Input: part model. Units: mm. Frame: model coordinates. Face numbers are marked on the shaded views. Round coordinates to 2 decimals unless told otherwise and drop trailing zeros. Order: outer loops, then holes, each group sorted by start corner. A loop starts at its lowest first (then second) coordinate and runs counter-clockwise, first axis right, second up. Notation, with made-up numbers: (76.25, 21.5) -> (92.25, 21.5) arc R31 ccw to (92.25, 56.5) -> close; hole circle Ø11 at (10, 16). An arc over 180 degrees is marked (long way). Use a Markdown table: item, result.
from build123d import *

# Parameters (mm, degrees)
SKETCH001_R      = 1.5875
EXTRUDE001_DEPTH = 7.62
SKETCH_R         = 3.556
EXTRUDE_DEPTH    = 3.81
BOX_W            = 60.325
BOX_H            = 45.72
BOX_DEPTH        = 6.35
THICKNESS_T      = -2.54
FILLET_R         = 3.56
FILLET001_R      = 6.1


with BuildPart() as extrude001:
    # Sketch001 (on Face9 of Extrude) → Extrude001 (new body)
    with BuildSketch(Plane.XY.offset(6.35)):
        with Locations((6.1, 39.62)):
            Circle(SKETCH001_R)
        with Locations((54.225, 39.62)):
            Circle(SKETCH001_R)
        with Locations((54.225, 6.1)):
            Circle(SKETCH001_R)
        with Locations((6.1, 6.1)):
            Circle(SKETCH001_R)
    extrude(amount=-EXTRUDE001_DEPTH)


with BuildPart() as extrude_body:
    # Sketch (on Face19 of Fillet001) → Extrude (new body)
    with BuildSketch(Plane.XY.offset(2.54)):
        with Locations((6.1, 39.62)):
            Circle(SKETCH_R)
        with Locations((54.225, 39.62)):
            Circle(SKETCH_R)
        with Locations((54.225, 6.1)):
            Circle(SKETCH_R)
        with Locations((6.1, 6.1)):
            Circle(SKETCH_R)
    extrude(amount=EXTRUDE_DEPTH)


with BuildPart() as cut:
    # Box → Box (new body)
    with BuildSketch(Plane.XY):
        with Locations((30.1625, 22.86)):
            Rectangle(BOX_W, BOX_H)
    extrude(amount=BOX_DEPTH)

    # Thickness
    thickness_openings = [cut.faces().sort_by_distance(p)[0] for p in [
        (30.1625, 22.86, 6.35),
    ]]
    offset(amount=THICKNESS_T, openings=thickness_openings, kind=Kind.INTERSECTION)

    # Fillet
    fillet_edges = [cut.edges().sort_by_distance(p)[0] for p in [
        (2.54, 2.54, 4.445),
        (2.54, 43.18, 4.445),
        (57.785, 2.54, 4.445),
        (57.785, 43.18, 4.445),
    ]]
    fillet(fillet_edges, radius=FILLET_R)

    # Fillet001
    fillet001_edges = [cut.edges().sort_by_distance(p)[0] for p in [
        (0, 0, 3.175),
        (0, 45.72, 3.175),
        (60.325, 0, 3.175),
        (60.325, 45.72, 3.175),
    ]]
    fillet(fillet001_edges, radius=FILLET001_R)

    # Fusion: union Extrude body
    add(extrude_body.part)

    # Cut: cut Extrude001
    add(extrude001.part, mode=Mode.SUBTRACT)


solid = cut.part
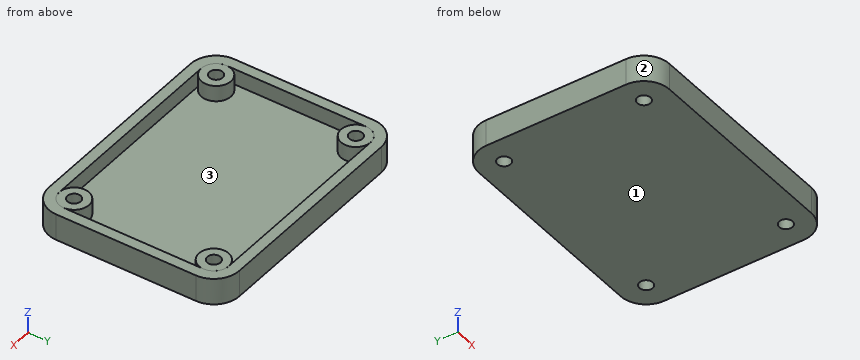
1) Cut plane A-A on z = 4.5. Count the separate pieces of the cut face and the enclosed holes in it, and give its area (3 significant figures).
Results found:
| item | result |
|---|---|
| separate pieces | 5 |
| enclosed holes | 5 |
| area | 619 mm² |
2) Cut plane C-C on y = 27. Return loops of the section in (x, z) (3 decimals), and give its area (3 significant figures).
Results found:
| item | result |
|---|---|
| outline | (0, 0) -> (60.325, 0) -> (60.325, 6.35) -> (57.785, 6.35) -> (57.785, 2.54) -> (2.54, 2.54) -> (2.54, 6.35) -> (0, 6.35) -> close |
| area | 173 mm² |
3) Pin query (flat end, axial travel): pin 1 Ø1.9 at (x, y) = (6.1, 39.62) entering from -Z; pin 2 Ø5 at (x, y) = (21.5, 25) entering from +Z; pin 3 Ø4 at (x, y) = (6.1, 6.1) entering from +Z. Return the tip coordinate at first contact, or that it passes through.
Results found:
| item | result |
|---|---|
| pin 1 | passes through |
| pin 2 | stops at z = 2.54 |
| pin 3 | stops at z = 6.35 |
4) Cut plane D-D on x = 44. Return loops of the section in (y, z).
Results found:
| item | result |
|---|---|
| outline | (0, 0) -> (45.72, 0) -> (45.72, 6.35) -> (43.18, 6.35) -> (43.18, 2.54) -> (2.54, 2.54) -> (2.54, 6.35) -> (0, 6.35) -> close |
5) Line query: L1, parallel to Y at x = 6.1, z = 2.25; L2, parallel to Y at x = 15.5, z = 3; L3, parallel to Z at x = 38.5, y = 23.5. Output: solid intervals per line, ascending. Write a range as [from, to].
Results found:
| item | result |
|---|---|
| L1 | y = [0, 4.51], [7.69, 38.03], [41.21, 45.72] |
| L2 | y = [0, 2.54], [43.18, 45.72] |
| L3 | z = [0, 2.54] |
6) Cut plane B-B on z = 1.25. Return loops of the section in (x, y) (1 decimal), and give its area (3 significant figures).
Results found:
| item | result |
|---|---|
| outline | (0, 6.1) arc R6.1 ccw to (6.1, 0) -> (54.2, 0) arc R6.1 ccw to (60.3, 6.1) -> (60.3, 39.6) arc R6.1 ccw to (54.2, 45.7) -> (6.1, 45.7) arc R6.1 ccw to (0, 39.6) -> close; hole circle Ø3.2 at (6.1, 6.1); hole circle Ø3.2 at (6.1, 39.6); hole circle Ø3.2 at (54.2, 6.1); hole circle Ø3.2 at (54.2, 39.6) |
| area | 2,690 mm² |
7) Pull-direction query (X, two-part tool) for the marked faces 1, 2 and 3; classes: +X half, -X half, draft (parallel to the pull), parting line (faces both ways), or undercut.
Results found:
| item | result |
|---|---|
| face 1 | draft |
| face 2 | -X half |
| face 3 | undercut |
